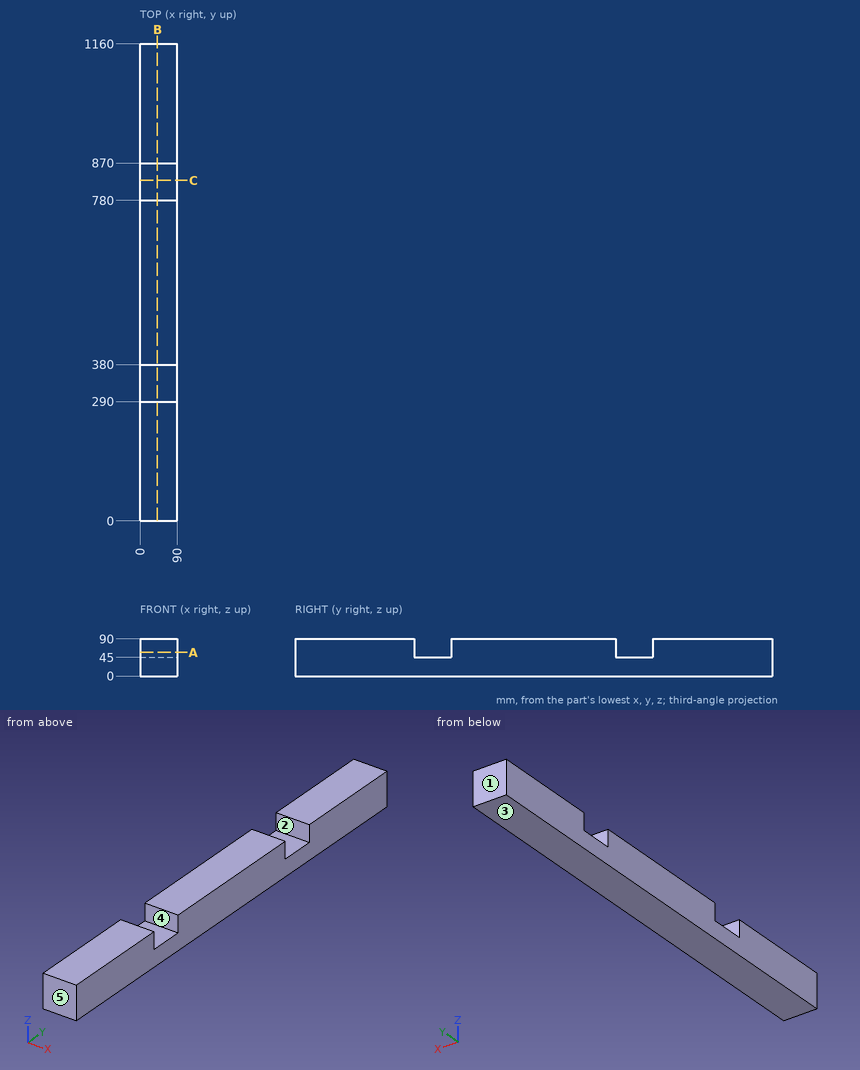
For this review, use the dimensioned drawing (mm, ordinates from the lowest corner) and the shaded views. A direction names the side the tool comes from. Coordinates: 2 decimals unless noted, no trailing zeros. Loops run counter-clockwise (first coordinate to the right, second up) from the corner with the lowest first, then second, coordinate; pieces in that order, holes last. Notation, with made-up numbers: (-13, 5.5) - (35, 5.5) arc R26 ccw to (35, 27.5) - close; hole circle Ø11 at (-26.5, 4). An arc over 180 degrees is marked (long way). Use one line per item in the form item = value. Start each with the question number.
1) To check wall thickness, follow probe 1 along Y at (x, z) = (17.5, 81.5); probe 2 along Z at (x, y) = (65, 784.5). State the ranges of each line that lie inside material, in increasing order. Write a range as from..to.
2) Draft analysis for pull direction Y (two halves, no side actions). For the marked faces 1, 2 and 3, state which applies: released by +Y, released by -Y, zero draft, split by the parting line, or undercut.
3) Take a section at A-A (z = 57.5). State the section outline as (x, y) points, plus the area to 3 significant figures.
4) Take a section at C-C (y = 828.5). State the section outline as (x, z) points.
5) For the marked faces 4 and 5, list the 3-axis set-ups (+Z, -Z, +X, -X, +Y, -Y) from which the entire face can be reached by the end or side of a thin tool; tool diameter is ignored.
6) Take a section at B-B (x = 42.5). State the section outline as (y, z) points, plus the area to 3 significant figures.
From the geometry:
q1.probe_1 = 0..290, 380..780, 870..1160
q1.probe_2 = 0..45
q2.face_1 = released by +Y
q2.face_2 = undercut
q2.face_3 = zero draft
q3.outline = (0, 0) - (90, 0) - (90, 290) - (0, 290) - close; (0, 380) - (90, 380) - (90, 780) - (0, 780) - close; (0, 870) - (90, 870) - (90, 1160) - (0, 1160) - close
q3.area = 88,200 mm2
q4.outline = (0, 0) - (90, 0) - (90, 45) - (0, 45) - close
q5.face_4 = +Z, +X, -X
q5.face_5 = +Z, -Z, +X, -X, -Y
q6.outline = (0, 0) - (1160, 0) - (1160, 90) - (870, 90) - (870, 45) - (780, 45) - (780, 90) - (380, 90) - (380, 45) - (290, 45) - (290, 90) - (0, 90) - close
q6.area = 96,300 mm2
